```python
from build123d import *

# Parameters (mm, degrees)
SKETCH1_W           = 25.780000002
SKETCH1_H           = 12.954026584
SKETCH1_R           = 3.025
BOSS_EXTRUDE1_DEPTH = 56.59882
FILLET2_R           = 2.54


with BuildPart() as part:
    # Sketch1 → Boss-Extrude1 (new body)
    with BuildSketch(Plane.XY):
        with Locations((-6.540000001, 85.048986708)):
            Rectangle(SKETCH1_W, SKETCH1_H)
        with Locations((0, 84.921973416)):
            Circle(SKETCH1_R, mode=Mode.SUBTRACT)
    extrude(amount=BOSS_EXTRUDE1_DEPTH)

    # Fillet2
    fillet2_edges = [part.edges().sort_by_distance(p)[0] for p in [
        (-19.430000002, 91.526, 28.29941),
        (6.35, 91.526, 28.29941),
        (6.35, 78.571973416, 28.29941),
        (-19.430000002, 78.571973416, 28.29941),
    ]]
    fillet(fillet2_edges, radius=FILLET2_R)


solid = part.part
```
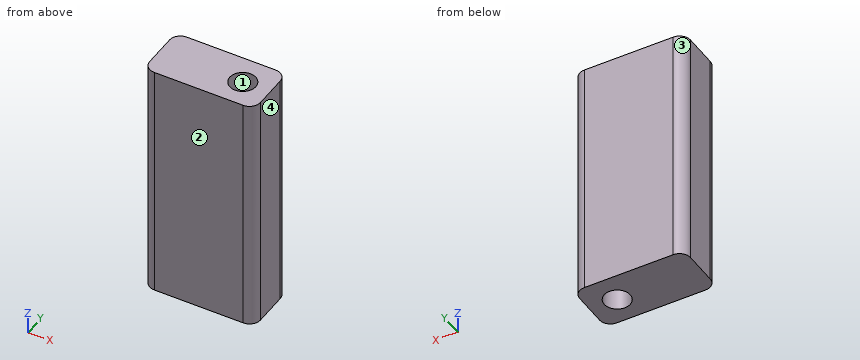
Work out the finished part from the listing and answer in its coordinate system (mm). Face numbers are marked on the shaded views. Round coordinates to 2 decimals unless told otherwise and drop trailing zeros. Write each loop counter-clockwise with the first axis right and the second up, starting at its lowest first coordinate (ties: lowest second). Pieces come first, ordered by that corner, then holes. Notation, with made-up numbers: (-2.75, 77.25) -> (5.25, 77.25) arc R24 cw to (5.25, 100.25) -> close; hole circle Ø1 at (-26, 65). An arc over 180 degrees is marked (long way). Write each question's results on one line, items separated by ' | '.
Q1. Section C-C, the plane z = 11 is taken. Write down the section's boundary in (x, y) (3 decimals).
Data:
outline: (-19.43, 81.112) arc R2.54 ccw to (-16.89, 78.572) -> (3.81, 78.572) arc R2.54 ccw to (6.35, 81.112) -> (6.35, 88.986) arc R2.54 ccw to (3.81, 91.526) -> (-16.89, 91.526) arc R2.54 ccw to (-19.43, 88.986) -> close; hole circle Ø6.05 at (0, 84.922)
Q2. Section A-A, the plane x = 0 is taken. Write down the section's boundary in (y, z).
Data:
outline: (78.57, 0) -> (81.9, 0) -> (81.9, 56.6) -> (78.57, 56.6) -> close; (87.95, 0) -> (91.53, 0) -> (91.53, 56.6) -> (87.95, 56.6) -> close
Q3. Section B-B, the plane y = 82.5 is taken. Write down the section's boundary in (x, z), then the cut area to 3 significant figures.
Data:
outline: (-19.43, 0) -> (-1.81, 0) -> (-1.81, 56.6) -> (-19.43, 56.6) -> close; (1.81, 0) -> (6.35, 0) -> (6.35, 56.6) -> (1.81, 56.6) -> close | area: 1,250 mm^2
Q4. Straight lines are drawn through the part: line 1 along X through (y, z) = (85.25, 4); line 2 along Y through (x, z) = (0, 32); line 3 along X through (y, z) = (84, 37). For each, find the intervals that lie inside material, in ascending order. Write a range as [from, to].
Data:
line 1: [-19.43, -3.01], [3.01, 6.35] | line 2: [78.57, 81.9], [87.95, 91.53] | line 3: [-19.43, -2.88], [2.88, 6.35]
Q5. Determine the mould class of the marked faces 1, 2, 3 and 4 for opening direction X: released by +X, released by -X, zero draft, split by the parting line, or undercut.
Data:
face 1: undercut | face 2: zero draft | face 3: released by -X | face 4: released by +X
Q6. Section D-D, the plane y = 90.75 is taken. Write down the section's boundary in (x, z), then the cut area to 3 significant figures.
Data:
outline: (-18.72, 0) -> (5.64, 0) -> (5.64, 56.6) -> (-18.72, 56.6) -> close | area: 1,380 mm^2
